Part model, mm, in its own coordinate system. Give positions to 0.01 mm unless a question says otherwise; leave off trailing zeros. Write each loop counter-clockwise with the first axis right and the second up, starting at its lowest first coordinate (ties: lowest second). Pieces come first, ordered by that corner, then holes. Notation, with made-up numbers: (3.5, 29) - (40.5, 29) arc R13 ccw to (40.5, 53) - close; hole circle Ø10 at (56, 11). An arc over 180 degrees is marked (long way). Answer as a JSON object with one key per item and string values. Group by question number.
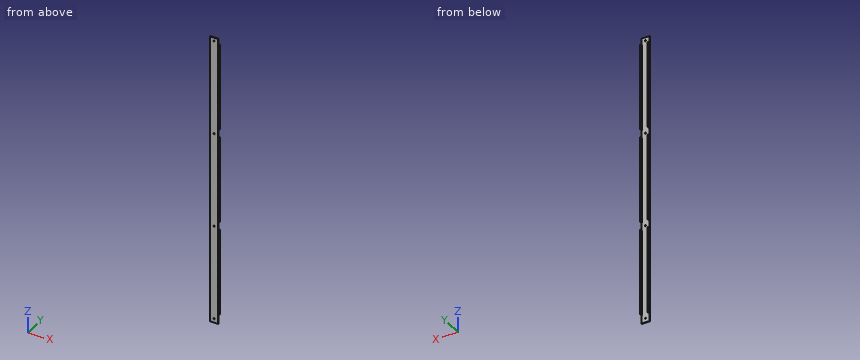
```python
from build123d import *

# Parameters (mm, degrees)
BOSS_EXTRUDE1_DEPTH = 1149.35
SKETCH2_W           = 132.323055729
SKETCH2_H           = 87.040299976
CUT_EXTRUDE1_DEPTH  = 9.525
SKETCH3_W           = 31.75
SKETCH3_H           = 12.7
CUT_EXTRUDE2_DEPTH  = 1150.858589132
SKETCH4_W           = 31.75
SKETCH4_H           = 12.7
CUT_EXTRUDE3_DEPTH  = 1150.858589132
SKETCH5_W           = 31.75
SKETCH5_H           = 12.7
CUT_EXTRUDE4_DEPTH  = 1150.858589132
CUT_EXTRUDE5_REACH  = 1151.828
SKETCH6_R           = 2.413


with BuildPart() as part:
    # Sketch1 → Boss-Extrude1 (new body)
    with BuildSketch(Plane.XY):
        Polygon((3.175, 3.175), (3.175, 12.7), (0, 12.7), (0, 0), (31.75, 0), (31.75, 12.7), (28.575, 12.7), (28.575, 3.175), align=None)
    extrude(amount=BOSS_EXTRUDE1_DEPTH)

    # Sketch2 → Cut-Extrude1 (cut)
    with BuildSketch(Plane(origin=(0, 3.175, 0), x_dir=(1, 0, 0), z_dir=(0, 1, 0))):
        with Locations((4.885698681, 11.770149988)):
            Rectangle(SKETCH2_W, SKETCH2_H)
    extrude(amount=CUT_EXTRUDE1_DEPTH, mode=Mode.SUBTRACT)

    # Sketch3 → Cut-Extrude2 (cut, through all)
    with BuildSketch(Plane.ZY):
        with Locations((389.255, 9.525)):
            Rectangle(SKETCH3_W, SKETCH3_H)
    extrude(amount=-CUT_EXTRUDE2_DEPTH, mode=Mode.SUBTRACT)

    # Sketch4 → Cut-Extrude3 (cut, through all)
    with BuildSketch(Plane.ZY):
        with Locations((762.635, 9.525)):
            Rectangle(SKETCH4_W, SKETCH4_H)
    extrude(amount=-CUT_EXTRUDE3_DEPTH, mode=Mode.SUBTRACT)

    # Sketch5 → Cut-Extrude4 (cut, through all)
    with BuildSketch(Plane.ZY):
        with Locations((1136.015, 9.525)):
            Rectangle(SKETCH5_W, SKETCH5_H)
    extrude(amount=-CUT_EXTRUDE4_DEPTH, mode=Mode.SUBTRACT)

    # Sketch6 → Cut-Extrude5 (cut, up to next)
    with BuildSketch(Plane(origin=(0, 3.175, 0), x_dir=(1, 0, 0), z_dir=(0, 1, 0)), mode=Mode.PRIVATE) as cut_extrude5_sk1:
        with Locations(Location((15.875, -15.875, 0), (0, 0, 270))):
            Circle(SKETCH6_R)
    cut_extrude5_tool1 = extrude(cut_extrude5_sk1.sketch, amount=-CUT_EXTRUDE5_REACH, mode=Mode.PRIVATE) & part.part
    # Sketch6 → Cut-Extrude5 (cut, up to next)
    with BuildSketch(Plane(origin=(0, 3.175, 0), x_dir=(1, 0, 0), z_dir=(0, 1, 0)), mode=Mode.PRIVATE) as cut_extrude5_sk2:
        with Locations(Location((15.875, -389.255, 0), (0, 0, 270))):
            Circle(SKETCH6_R)
    cut_extrude5_tool2 = extrude(cut_extrude5_sk2.sketch, amount=-CUT_EXTRUDE5_REACH, mode=Mode.PRIVATE) & part.part
    # Sketch6 → Cut-Extrude5 (cut, up to next)
    with BuildSketch(Plane(origin=(0, 3.175, 0), x_dir=(1, 0, 0), z_dir=(0, 1, 0)), mode=Mode.PRIVATE) as cut_extrude5_sk3:
        with Locations(Location((15.875, -762.635, 0), (0, 0, 270))):
            Circle(SKETCH6_R)
    cut_extrude5_tool3 = extrude(cut_extrude5_sk3.sketch, amount=-CUT_EXTRUDE5_REACH, mode=Mode.PRIVATE) & part.part
    # Sketch6 → Cut-Extrude5 (cut, up to next)
    with BuildSketch(Plane(origin=(0, 3.175, 0), x_dir=(1, 0, 0), z_dir=(0, 1, 0)), mode=Mode.PRIVATE) as cut_extrude5_sk4:
        with Locations(Location((15.875, -1136.015, 0), (0, 0, 270))):
            Circle(SKETCH6_R)
    cut_extrude5_tool4 = extrude(cut_extrude5_sk4.sketch, amount=-CUT_EXTRUDE5_REACH, mode=Mode.PRIVATE) & part.part
    add(cut_extrude5_tool1.solids().sort_by_distance((15.875, 3.175, 15.875))[0], mode=Mode.SUBTRACT)
    add(cut_extrude5_tool2.solids().sort_by_distance((15.875, 3.175, 389.255))[0], mode=Mode.SUBTRACT)
    add(cut_extrude5_tool3.solids().sort_by_distance((15.875, 3.175, 762.635))[0], mode=Mode.SUBTRACT)
    add(cut_extrude5_tool4.solids().sort_by_distance((15.875, 3.175, 1136.015))[0], mode=Mode.SUBTRACT)


solid = part.part
```
1) Band-saw the part on B-B (z = 1007). List the corners of the cut face in (x, y) (3 decimals), plus the area to 3 significant figures.
2) Probe line 1 (X direction, y = 10.25, z = 940.5) (3 decimals); line 2 (Y direction, x = 9, z = 347) (3 decimals). List the from-to ranges inside material, lowest first.
3) Band-saw the part on C-C (x = 23.5). List the corners of the cut face in (y, z) (3 decimals).
4) Band-saw the part on A-A (y = 7.75). List the corners of the cut face in (x, z) (3 decimals), plus the area to 3 significant figures.
5) Drop flat-ended pins along their axis: P1, Ø3.5, axis at x = 29.5, y = 9, coming from the +Z side; P2, Ø2.5, axis at x = 1, y = 7.5, coming from the -Z side; P3, Ø16, axis at x = 19, z = 758.5, coming from the +Y side (3 decimals). Give the stop position or say it passes through.
Verdict:
{
 "1": {"outline": "(0, 0) - (31.75, 0) - (31.75, 12.7) - (28.575, 12.7) - (28.575, 3.175) - (3.175, 3.175) - (3.175, 12.7) - (0, 12.7) - close", "area": "161 mm2"},
 "2": {"line 1": "0 to 3.175, 28.575 to 31.75", "line 2": "0 to 3.175"},
 "3": {"outline": "(0, 0) - (3.175, 0) - (3.175, 1149.35) - (0, 1149.35) - close"},
 "4": {"outline": "(0, 31.75) - (3.175, 31.75) - (3.175, 373.38) - (0, 373.38) - close; (0, 405.13) - (3.175, 405.13) - (3.175, 746.76) - (0, 746.76) - close; (0, 778.51) - (3.175, 778.51) - (3.175, 1120.14) - (0, 1120.14) - close; (28.575, 31.75) - (31.75, 31.75) - (31.75, 373.38) - (28.575, 373.38) - close; (28.575, 405.13) - (31.75, 405.13) - (31.75, 746.76) - (28.575, 746.76) - close; (28.575, 778.51) - (31.75, 778.51) - (31.75, 1120.14) - (28.575, 1120.14) - close", "area": "6,510 mm2"},
 "5": {"P1": "z = 1120.14", "P2": "z = 31.75", "P3": "y = 3.175"}
}
